Part model, mm, in its own coordinate system. A direction names the side the tool comes from. Coordinates: 2 decimals unless noted, no trailing zeros. Order: outer loops, then holes, each group sorted by start corner. A loop starts at its lowest first (then second) coordinate and runs counter-clockwise, first axis right, second up. Notation, with made-up numbers: (37, 73) - (96, 73) arc R10 ccw to (96, 78) - close; hole circle Ø8 at (-13, 37). An arc over 180 degrees is marked (long way). Use a Markdown table: item, result. Add a question column.
1) Saw through at D-D on x = 13.5. List the corners of the cut face in (y, z).
2) Saw through at C-C on z = 6.25. List the corners of the cut face in (x, y).
3) Drop flat-ended pins along their axis: P1, Ø1.5, axis at y = 19.5, z = 6, coming from the -X side; P2, Ø1.2, axis at y = 23.5, z = 6, coming from the -X side; P3, Ø2, axis at y = 11, z = 6.5, coming from the -X side; P4, Ø1.5, axis at x = 4.5, y = 3, coming from the -Z side. Give the stop position or say it passes through.
4) Two-plate mould, pull along Y, no slides. Class faces 1 (the face through (-22.699, 0.285, 4.314)), 2 (the face through (0, 13, 0)), 3 (the face through (-4, 17, 1.5)): +Y half, -Y half, draft (parallel to the pull), parting line (faces both ways), or undercut.
5) Saw through at B-B on x = 5. List the corners of the cut face in (y, z), then the cut area to 4 significant figures.
6) Saw through at A-A on y = 8. List the corners of the cut face in (x, z), then the cut area to 3 significant figures.
7) Tool access for faces 4 (the face through (10, 15, 5)), 5 (the face through (7, 25, 5)), 6 (the face through (0.86, 12.1, 1.9)): list every direction of +Z, -Z, +X, -X, +Y, -Y with a clear straight run to the whole face (end or side of a thin tool).
8) Wall check: L1, parallel to Y at x = 5, z = 5.1; L2, parallel to Y at x = 12.5, z = 6.75; L3, parallel to X at y = 22, z = 4.5. Give the ranges that are in metal, low to high. Write a range as [from, to].
```python
from build123d import *

# Parameters (mm, degrees)
PAD098_DEPTH    = 2
PAD099_DEPTH    = 6.75
SKETCH137_W     = 2
SKETCH137_H     = 23
SKETCH137_W_2   = 21
SKETCH137_H_2   = 2
POCKET040_DEPTH = 1
SKETCH138_W     = 10
SKETCH138_H     = 10
PAD100_DEPTH    = 5
SKETCH139_R     = 2.5
POCKET041_DEPTH = 5
FILLET024_R     = 2.99
FILLET025_R     = 1
FILLET026_R     = 3


with BuildPart() as part:
    # Sketch135 → Pad098 (new body)
    with BuildSketch(Plane.XY):
        Polygon((-23, 18), (-23, 0), (0, 0), (0, 13), (23, 13), (23, 26), (-7, 26), (-9, 26), (-9, 21), (-13, 20), (-23, 20), align=None)
    extrude(amount=PAD098_DEPTH)

    # Sketch136 (on Face13 of Pad098) → Pad099 (join)
    with BuildSketch(Plane.XY.offset(2)):
        Polygon((-23, 0), (0, 0), (0, 13), (23, 13), (23, 26), (-9, 26), (-9, 21), (-13, 20), (-23, 20), (-23, 18), (-13, 18), (-7, 19), (-7, 25), (21, 25), (21, 15), (-2, 15), (-2, 2), (-23, 2), align=None)
    extrude(amount=PAD099_DEPTH)

    # Sketch137 (on Face7 of Pad099) → Pocket040 (cut)
    with BuildSketch(Plane.XY.offset(2)):
        with Locations((-6, 13.5)):
            Rectangle(SKETCH137_W, SKETCH137_H)
        with Locations((6.5, 17)):
            Rectangle(SKETCH137_W_2, SKETCH137_H_2)
    extrude(amount=-POCKET040_DEPTH, mode=Mode.SUBTRACT)

    # Sketch138 (on Face18 of Pocket040) → Pad100 (join)
    with BuildSketch(Plane.XY.offset(8.75)):
        with Locations((5, 8)):
            Rectangle(SKETCH138_W, SKETCH138_H)
    extrude(amount=-PAD100_DEPTH)

    # Sketch139 (on Face29 of Pad100) → Pocket041 (cut)
    with BuildSketch(Plane.XY.offset(8.75)):
        with Locations((5, 8)):
            Circle(SKETCH139_R)
    extrude(amount=-POCKET041_DEPTH, mode=Mode.SUBTRACT)

    # Fillet024
    fillet024_edges = [part.edges().sort_by_distance(p)[0] for p in [
        (10, 3, 6.25),
    ]]
    fillet(fillet024_edges, radius=FILLET024_R)

    # Fillet025
    fillet025_edges = [part.edges().sort_by_distance(p)[0] for p in [
        (23, 13, 1),
        (23, 13, 5.375),
        (0, 0, 5.375),
        (0, 0, 1),
        (-23, 0, 5.375),
        (-23, 0, 1),
        (23, 26, 1),
        (23, 26, 5.375),
        (-23, 20, 1),
        (-23, 20, 5.375),
        (-9, 26, 1),
        (-9, 26, 5.375),
    ]]
    fillet(fillet025_edges, radius=FILLET025_R)

    # Fillet026
    fillet026_edges = [part.edges().sort_by_distance(p)[0] for p in [
        (0, 13, 2.875),
        (0, 13, 1),
    ]]
    fillet(fillet026_edges, radius=FILLET026_R)


solid = part.part
```
Results are:
| question | item | result |
|---|---|---|
| 1 | outline | (13, 0) - (26, 0) - (26, 8.75) - (25, 8.75) - (25, 2) - (18, 2) - (18, 1) - (16, 1) - (16, 2) - (15, 2) - (15, 8.75) - (13, 8.75) - close |
| 2 | outline | (-23, 1) arc R1 ccw to (-22, 0) - (-1, 0) arc R1 ccw to (0, 1) - (0, 3) - (7.01, 3) arc R2.99 ccw to (10, 5.99) - (10, 13) - (22, 13) arc R1 ccw to (23, 14) - (23, 25) arc R1 ccw to (22, 26) - (-8, 26) arc R1 ccw to (-9, 25) - (-9, 21) - (-13, 20) - (-22, 20) arc R1 ccw to (-23, 19) - (-23, 18) - (-13, 18) - (-7, 19) - (-7, 25) - (21, 25) - (21, 15) - (-2, 15) - (-2, 2) - (-23, 2) - close; hole circle Ø5 at (5, 8) |
| 3 | P1 | x = -23 |
| 3 | P2 | x = -9 |
| 3 | P3 | x = -2 |
| 3 | P4 | z = 3.75 |
| 4 | face 1 | -Y half |
| 4 | face 2 | draft |
| 4 | face 3 | undercut |
| 5 | outline | (3, 3.75) - (5.5, 3.75) - (5.5, 8.75) - (3, 8.75) - close; (10.5, 3.75) - (13, 3.75) - (13, 0) - (26, 0) - (26, 8.75) - (25, 8.75) - (25, 2) - (18, 2) - (18, 1) - (16, 1) - (16, 2) - (15, 2) - (15, 8.75) - (10.5, 8.75) - close |
| 5 | area | 69.25 mm2 |
| 6 | outline | (-23, 0) - (0, 0) - (0, 3.75) - (2.5, 3.75) - (2.5, 8.75) - (-2, 8.75) - (-2, 2) - (-5, 2) - (-5, 1) - (-7, 1) - (-7, 2) - (-23, 2) - close; (7.5, 3.75) - (10, 3.75) - (10, 8.75) - (7.5, 8.75) - close |
| 6 | area | 82.5 mm2 |
| 7 | face 4 | +Z, -X |
| 7 | face 5 | +Z |
| 7 | face 6 | -Z, +X, -Y |
| 8 | L1 | [3, 5.5], [10.5, 15], [25, 26] |
| 8 | L2 | [13, 15], [25, 26] |
| 8 | L3 | [-9, -7], [21, 23] |
